from build123d import *

# Parameters (mm, degrees)
F1_DEPTH = 95.25
F2_R     = 6.35
F3_DEPTH = 25.4
F4_R     = 6.35
F5_DEPTH = 6.35
F7_DEPTH = 25.4


with BuildPart() as f1:
    # F0 (on Top) → F1 (new body)
    with BuildSketch(Plane.XY):
        with BuildLine():
            Line((9.525, 0), (6.35, 0))
            ThreePointArc((6.35, 0), (-6.2239381909, 1.2590049228), (5.8507579856, -2.4680216762))
            Line((5.8507579856, -2.4680216762), (6.35, -2.4680216762))
            Line((6.35, -2.4680216762), (6.35, -146.05))
            Line((6.35, -146.05), (9.525, -146.05))
            Line((9.525, -146.05), (9.525, 0))
        make_face()
    extrude(amount=F1_DEPTH)

    # F2 (on face) → F3 (join)
    with BuildSketch(Plane.XY.offset(95.25)):
        Circle(F2_R)
    extrude(amount=F3_DEPTH)

    # F4 (on face) → F5 (join)
    with BuildSketch(Plane(origin=(0, 0, 0), x_dir=(1, 0, 0), z_dir=(0, 0, -1))):
        Circle(F4_R)
    extrude(amount=F5_DEPTH)

    # F6 (on face) → F7 (cut)
    with BuildSketch(Plane.YZ.offset(9.525)):
        with BuildLine():
            ThreePointArc((-146.05, 92.075), (-145.1200640303, 94.3200640303), (-142.875, 95.25))
            Line((-142.875, 95.25), (-146.05, 95.25))
            Line((-146.05, 95.25), (-146.05, 92.075))
        make_face()
        with BuildLine():
            ThreePointArc((-142.875, 0), (-145.1200640303, 0.9299359697), (-146.05, 3.175))
            Line((-146.05, 3.175), (-146.05, 0))
            Line((-146.05, 0), (-142.875, 0))
        make_face()
    extrude(amount=-F7_DEPTH, mode=Mode.SUBTRACT)


solid = f1.part
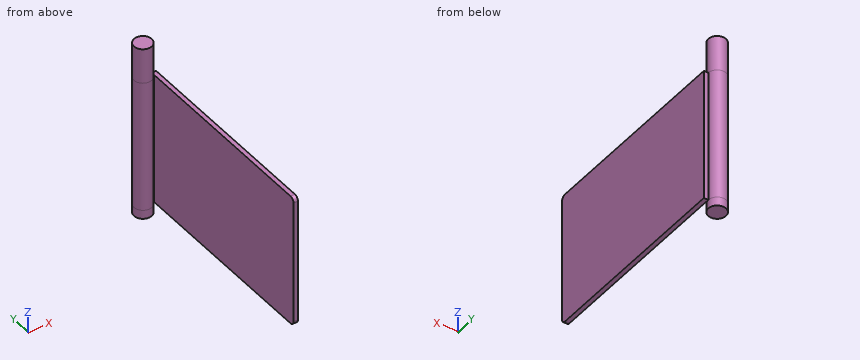
Read the model definition and answer for the solid it produces. Units are mm, in the model's axes. Coordinates: 2 decimals unless noted, no trailing zeros. Loops run counter-clockwise (first coordinate to the right, second up) from the corner with the lowest first, then second, coordinate; pieces in that order, holes last. Notation, with made-up numbers: (-11, -28.5) - (19, -28.5) arc R27 ccw to (19, 3.5) - close; hole circle Ø9 at (76.25, 36). An arc over 180 degrees is marked (long way). Answer in a Markdown table with one row per item.
Q1. Given P1, Ø6, axis at x = 1, z = 15.5, coming from the -Y side; P2, Ø1, axis at y = -57.5, z = 77.5, coming from the -X side; P3, Ø1.8, axis at x = 8, y = -59.5, coming from the -Z side, each flat-ended and moving along its own axis, determine where each tip first touches the part or whether it passes through.
Here are the results:
| item | result |
|---|---|
| P1 | stops at y = -6.35 |
| P2 | stops at x = 6.35 |
| P3 | stops at z = 0 |
Q2. Find section C-C on y = -86.5. Write down the section's boundary in (x, z) (3 decimals), plus the area to 3 significant figures.
Here are the results:
| item | result |
|---|---|
| outline | (6.35, 0) - (9.525, 0) - (9.525, 95.25) - (6.35, 95.25) - close |
| area | 302 mm^2 |
Q3. Straight lines are drawn through the part: line 1 along X through (y, z) = (-37, 27) (3 decimals); line 2 along Y through (x, z) = (8.25, 23); line 3 along Y through (x, z) = (0, 97). For each, find the intervals that lie inside material, in ascending order. Write a range as [from, to].
Here are the results:
| item | result |
|---|---|
| line 1 | x = [6.35, 9.525] |
| line 2 | y = [-146.05, 0] |
| line 3 | y = [-6.35, 6.35] |
Q4. Find section B-B on z = 90. Write down the section's boundary in (x, y) (3 decimals).
Here are the results:
| item | result |
|---|---|
| outline | (5.851, -2.468) - (6.35, -2.468) - (6.35, -146.05) - (9.525, -146.05) - (9.525, 0) - (6.35, 0) arc R6.35 ccw (long way) to start |
Q5. Find section A-A on x = 0. Write down the section's boundary in (y, z).
Here are the results:
| item | result |
|---|---|
| outline | (-6.35, -6.35) - (6.35, -6.35) - (6.35, 120.65) - (-6.35, 120.65) - close |
